from build123d import *

# Parameters (mm, degrees)
SKETCH_12_R         = 2.75
EXTRUDE_3_DEPTH     = 2
SKETCH_13_R         = 1.5
EXTRUDE_4_DEPTH     = 7
SKETCH_20_W         = 6.034936197
SKETCH_20_H         = 0.8
CUT_EXTRUDE_8_DEPTH = 0.95
CHAMFER_1_SIZE      = 0.5


with BuildPart() as part:
    # Эскиз12 → Вытянуть3 (new body)
    with BuildSketch(Plane.XY):
        Circle(SKETCH_12_R)
    extrude(amount=EXTRUDE_3_DEPTH)

    # Эскиз13 → Вытянуть4 (add)
    with BuildSketch(Plane(origin=(0, 0, 0), x_dir=(-1, 0, 0), z_dir=(0, 0, -1))):
        with Locations(Location((0, 0, 0), (0, 0, 180))):
            Circle(SKETCH_13_R)
    extrude(amount=EXTRUDE_4_DEPTH)

    # Эскиз20 → Вырез-Вытянуть8 (cut)
    with BuildSketch(Plane.XY.offset(2)):
        with Locations((-0.014122315, 0)):
            Rectangle(SKETCH_20_W, SKETCH_20_H)
    extrude(amount=-CUT_EXTRUDE_8_DEPTH, mode=Mode.SUBTRACT)

    # Фаска1
    chamfer_1_edges = [part.edges().sort_by_distance(p)[0] for p in [
        (-1.5, 0, -7),
    ]]
    chamfer(chamfer_1_edges, length=CHAMFER_1_SIZE)


solid = part.part
CAD build for the part. Positions are in the model's coordinates, mm. A direction names the side the tool comes from. Give positions to 0.01 mm unless a question says otherwise; leave off trailing zeros. Write each loop counter-clockwise with the first axis right and the second up, starting at its lowest first coordinate (ties: lowest second). Pieces come first, ordered by that corner, then holes. Notation, with made-up numbers: (7, 61.25) - (59, 61.25) arc R23 ccw to (59, 89.25) - close; hole circle Ø4 at (82.25, -26.75). An arc over 180 degrees is marked (long way). Put each result on its own line as item: value.
(1) Saw through at A-A (y = 0). List the corners of the cut face in (x, z).
Working result:
outline: (-2.75, 0) - (-1.5, 0) - (-1.5, -6.5) - (-1, -7) - (1, -7) - (1.5, -6.5) - (1.5, 0) - (2.75, 0) - (2.75, 1.05) - (-2.75, 1.05) - close
(2) Saw through at B-B (x = 0). List the corners of the cut face in (y, z).
Working result:
outline: (-2.75, 0) - (-1.5, 0) - (-1.5, -6.5) - (-1, -7) - (1, -7) - (1.5, -6.5) - (1.5, 0) - (2.75, 0) - (2.75, 2) - (0.4, 2) - (0.4, 1.05) - (-0.4, 1.05) - (-0.4, 2) - (-2.75, 2) - close
(3) Pull direction Y, two halves, no side cores. Call faces 1 (the flat face through (0, -0.4, 1.5)), 2 (the flat face through (0, 0, -7)), 3 (the cylindrical face through (1.43, -0.45, -3.2)), 4 (the flat face through (0, 0.4, 1.5)): released by +Y, released by -Y, zero draft, split by the parting line, or undercut.
Working result:
face 1: undercut
face 2: zero draft
face 3: split by the parting line
face 4: undercut
(4) Drop flat-ended pins along their axis: pin 1 Ø0.8 at (x, z) = (-0.5, 1.5) entering from -Y; pin 2 Ø2 at (y, z) = (1, -6) entering from -X; pin 3 Ø3 at (x, z) = (0.5, -3) entering from +Y. Give the stop position or say it passes through.
Working result:
pin 1: y = -2.75
pin 2: x = -1.5
pin 3: y = 1.5
(5) Saw through at D-D (x = 1.85). List the corners of the cut face in (y, z), then the cut area to 3 significant figures.
Working result:
outline: (-2.03, 0) - (2.03, 0) - (2.03, 2) - (0.4, 2) - (0.4, 1.05) - (-0.4, 1.05) - (-0.4, 2) - (-2.03, 2) - close
area: 7.38 mm^2
(6) Saw through at C-C (z = -5). List the corners of the cut face in (x, y), then the cut area to 3 significant figures.
Working result:
outline: circle Ø3 at (0, 0)
area: 7.07 mm^2
(7) Tool access for faces 5 (the flat face through (0, 1, 2)), 6 (the flat face through (1.2, -1.2, 0)), 7 (the flat face through (0, 0, 1.05)): list every direction of +Z, -Z, +X, -X, +Y, -Y with a clear straight run to the whole face (end or side of a thin tool).
Working result:
face 5: +Z, +X, -X, +Y, -Y
face 6: -Z
face 7: +Z, +X, -X
(8) Wall check: L1, parallel to Z at x = 0.5, y = 2.1; L2, parallel to X at y = -2.35, z = 0.75; L3, parallel to Y at x = 0.65, z = -0.75. Give the ranges that are in metal, low to high.
Working result:
L1: 0 to 2
L2: -1.43 to 1.43
L3: -1.35 to 1.35
